from build123d import *

# Parameters (mm, degrees)
F0_R     = 11.005661
F0_R_2   = 7.5
F1_DEPTH = 8
F2_R     = 2


with BuildPart() as f1:
    # F0 (on Top) → F1 (new body)
    with BuildSketch(Plane.XY):
        with BuildLine():
            ThreePointArc((15.690977, 19.462612), (10.66965, 22.608816), (5.048904, 24.484864))
            ThreePointArc((5.048904, 24.484864), (-4.747707, 57.303658), (-9.009628, 23.32009))
            ThreePointArc((-9.009628, 23.32009), (-14.244984, 20.544596), (-18.680062, 16.614912))
            ThreePointArc((-18.680062, 16.614912), (-52.000278, 24.540194), (-24.700604, 3.857479))
            ThreePointArc((-24.700604, 3.857479), (-24.914634, -2.064221), (-23.728966, -7.869952))
            ThreePointArc((-23.728966, -7.869952), (-47.25257, -32.763464), (-15.690977, -19.462612))
            ThreePointArc((-15.690977, -19.462612), (-10.66965, -22.608816), (-5.048904, -24.484864))
            ThreePointArc((-5.048904, -24.484864), (4.747707, -57.303658), (9.009628, -23.32009))
            ThreePointArc((9.009628, -23.32009), (14.244984, -20.544596), (18.680062, -16.614912))
            ThreePointArc((18.680062, -16.614912), (52.000278, -24.540194), (24.700604, -3.857479))
            ThreePointArc((24.700604, -3.857479), (24.914634, 2.064221), (23.728966, 7.869952))
            ThreePointArc((23.728966, 7.869952), (47.25257, 32.763464), (15.690977, 19.462612))
        make_face()
        with Locations((-32.871353, -22.791975)):
            Circle(F0_R, mode=Mode.SUBTRACT)
        with Locations((3.302753, -39.863415)):
            Circle(F0_R, mode=Mode.SUBTRACT)
        with Locations((36.174106, -17.071439)):
            Circle(F0_R, mode=Mode.SUBTRACT)
        with Locations((-36.174106, 17.071439)):
            Circle(F0_R, mode=Mode.SUBTRACT)
        with Locations((-3.302753, 39.863415)):
            Circle(F0_R, mode=Mode.SUBTRACT)
        Circle(F0_R_2, mode=Mode.SUBTRACT)
        with Locations((32.871353, 22.791975)):
            Circle(F0_R, mode=Mode.SUBTRACT)
    extrude(amount=F1_DEPTH)

    # F2
    f2_edges = [f1.edges().sort_by_distance(p)[0] for p in [
        (15.690977, 19.462612, 4),
        (5.048904, 24.484864, 4),
        (-9.009628, 23.32009, 4),
        (-18.680062, 16.614912, 4),
        (24.700604, -3.857479, 4),
        (23.728966, 7.869952, 4),
        (18.680062, -16.614912, 4),
        (9.009628, -23.32009, 4),
        (-5.048904, -24.484864, 4),
        (-15.690977, -19.462612, 4),
        (-23.728966, -7.869952, 4),
        (-24.700604, 3.857479, 4),
    ]]
    fillet(f2_edges, radius=F2_R)


solid = f1.part
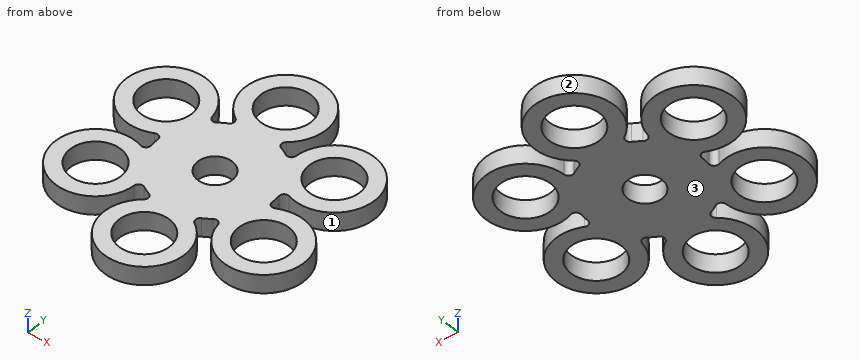
Source: CAD feature listing. Evaluate the final solid. Frame: model axes, mm. Face numbers are marked on the shaded views. Give positions to 0.01 mm unless a question says otherwise; leave off trailing zeros. Write each loop counter-clockwise with the first axis right and the second up, starting at its lowest first coordinate (ties: lowest second). Pieces come first, ordered by that corner, then holes. Notation, with made-up numbers: M 24,88.25 L 71,88.25 A18 ccw 71,102.25 Z; hole C 55,34.25 d4. An arc over 180 degrees is marked long. Answer as a JSON object with one key per item and string values.
Q1. Cut plane A-A, the plane x = 0. Return the cut outline in (y, z).
Geometry check:
{"outline": "M -57.05,0 L -50.36,0 L -50.36,8 L -57.05,8 Z; M -29.37,0 L -7.5,0 L -7.5,8 L -29.37,8 Z; M 7.5,0 L 29.37,0 L 29.37,8 L 7.5,8 Z; M 50.36,0 L 57.05,0 L 57.05,8 L 50.36,8 Z"}
Q2. Contact query for flat-ended pins moving along their axis: P1, Ø1.5, axis at x = 28, z = 7, coming from the -Y side; P2, Ø2, axis at x = -23.5, z = 2, coming from the +Y side; P3, Ø4, axis at x = 24, z = 6, coming from the +Y side; P4, Ø13.5, axis at x = 0, y = 0, coming from the -Z side. Output: stop coordinate, or through.
Geometry check:
{"P1": "stops at y = -32.92", "P2": "stops at y = 30.11", "P3": "stops at y = 38.89", "P4": "passes through"}
Q3. Cut plane B-B, the plane z = 5.5. Count the separate pieces of the cut face and the enclosed holes in it, then the cut area to 3 significant figures.
Geometry check:
{"separate pieces": "1", "enclosed holes": "7", "area": "5,170 mm^2"}
Q4. Ray query, line 1 along X through (y, z) = (33, 2); line 2 along X through (y, z) = (-40.5, 6.5); line 3 along Y through (x, z) = (-3.5, 1.5). Return the intervals inside material, ascending.
Geometry check:
{"line 1": "x = -43.42 to -28.93, -19.4 to -11.91, 5.3 to 12.8, 18.66 to 28.76, 36.98 to 47.09", "line 2": "x = -14.19 to -7.68, 14.29 to 20.79", "line 3": "y = -55.99 to -48.51, -31.21 to -6.63, 6.63 to 28.86, 50.87 to 57.36"}
Q5. Mould query, pull axis Y, two halves, no side actions, for the marked faces 1, 2 and 3. Classes: +Y half, -Y half, draft (parallel to the pull), parting line (faces both ways), or undercut.
Geometry check:
{"face 1": "undercut", "face 2": "undercut", "face 3": "draft"}
